For this review, take the finished solid that the model builds, in its own axes (mm). Face numbers are marked on the shaded views. A direction names the side the tool comes from. Round coordinates to 2 decimals unless told otherwise and drop trailing zeros. Write each loop counter-clockwise with the first axis right and the second up, starting at its lowest first coordinate (ties: lowest second). Pieces come first, ordered by that corner, then holes. Notation, with made-up numbers: (25.25, -13.75) -> (57.25, -13.75) arc R21 cw to (57.25, -2.75) -> close; hole circle Ø8 at (47.25, 79). An arc over 180 degrees is marked (long way). Answer as CSV lines item,"result". Start each with the question number.
Item 1: Take a section at B-B on z = 5.75. Give the boundary of the cut face in (x, y), then the cut area to 3 significant figures.
Item 2: Take a section at A-A on y = -2. Give the boundary of the cut face in (x, z).
Item 3: Mouldability with a two-part tool opening along Y and no side actions: class the marked faces 4, 5 and 6 as +Y half, -Y half, draft (parallel to the pull), parting line (faces both ways), or undercut.
Item 4: For pin 1 Ø1.7 at (x, y) = (-17, -1) entering from +Z; pin 2 Ø0.6 at (y, z) = (0, 9) entering from +X; pin 3 Ø4 at (x, y) = (-13, 2) entering from +Z, all flat-tipped, find the tip position at first contact; note any pin that passes through.
Item 5: Take a section at C-C on x = -17. Give the boundary of the cut face in (y, z).
Item 6: Machinability: for the marked faces 1, 2 and 3, which of the approach directions +Z, -Z, +X, -X, +Y, -Y give a long, thin tool a straight path to every point of the face, cutting with its end or side? Answer none if there is none.
Item 7: Wall thickness on probe 1 along Y at (x, z) = (17, 4.25); probe 2 along Y at (x, z) = (16.5, 3.5); probe 3 along Z at (x, y) = (-9.5, -1): over which ranges is each line inside the solid? List them lowest first. Write a range as from..to.
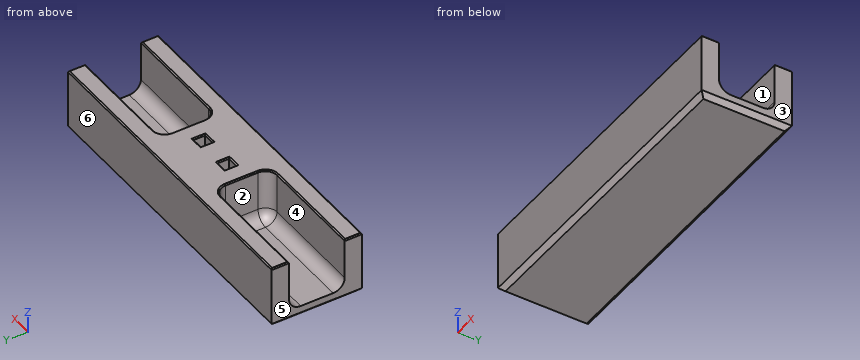
```python
from build123d import *

# Parameters (mm, degrees)
F0_W     = 55
F0_H     = 15.6
F1_DEPTH = 11
F2_W     = 2
F2_H     = 2
F3_DEPTH = 4
F4_W     = 20.27
F4_H     = 9.6
F5_DEPTH = 9
F6_R     = 2
F7_SIZE  = 0.2
F8_SIZE  = 0.8


with BuildPart() as f1:
    # F0 (on Top) → F1 (new body)
    with BuildSketch(Plane.XY):
        Rectangle(F0_W, F0_H)
    extrude(amount=F1_DEPTH)

    # F2 (on face) → F3 (cut)
    with BuildSketch(Plane.XY.offset(11)):
        with Locations((-3.23, 0)):
            Rectangle(F2_W, F2_H)
        with Locations((3.23, 0)):
            Rectangle(F2_W, F2_H)
    extrude(amount=-F3_DEPTH, mode=Mode.SUBTRACT)

    # F4 (on face) → F5 (cut)
    with BuildSketch(Plane.XY.offset(11)):
        with Locations((-17.365, 0)):
            Rectangle(F4_W, F4_H)
        with Locations((17.365, 0)):
            Rectangle(F4_W, F4_H)
    extrude(amount=-F5_DEPTH, mode=Mode.SUBTRACT)

    # F6
    f6_edges = [f1.edges().sort_by_distance(p)[0] for p in [
        (-7.23, 4.8, 6.5),
        (-17.365, 4.8, 2),
        (-7.23, 0, 2),
        (-17.365, -4.8, 2),
        (-7.23, -4.8, 6.5),
        (7.23, 0, 2),
        (7.23, 4.8, 6.5),
        (17.365, 4.8, 2),
        (17.365, -4.8, 2),
        (7.23, -4.8, 6.5),
    ]]
    fillet(f6_edges, radius=F6_R)

    # F7
    f7_edges = [f1.edges().sort_by_distance(p)[0] for p in [
        (-18.365, -4.8, 11),
        (-7.815786, -4.214214, 11),
        (-27.5, -6.3, 11),
        (-7.23, 0, 11),
        (0, -7.8, 11),
        (-7.815786, 4.214214, 11),
        (27.5, -6.3, 11),
        (-18.365, 4.8, 11),
        (18.365, -4.8, 11),
        (-27.5, 6.3, 11),
        (7.815786, -4.214214, 11),
        (0, 7.8, 11),
        (7.23, 0, 11),
        (27.5, 6.3, 11),
        (7.815786, 4.214214, 11),
        (18.365, 4.8, 11),
        (-2.23, 0, 11),
        (-3.23, -1, 11),
        (-3.23, 1, 11),
        (-4.23, 0, 11),
        (3.23, 1, 11),
        (4.23, 0, 11),
        (2.23, 0, 11),
        (3.23, -1, 11),
    ]]
    chamfer(f7_edges, length=F7_SIZE)

    # F8
    f8_edges = [f1.edges().sort_by_distance(p)[0] for p in [
        (27.5, 0, 0),
        (0, 7.8, 0),
        (-27.5, 0, 0),
        (0, -7.8, 0),
    ]]
    chamfer(f8_edges, length=F8_SIZE)


solid = f1.part
```
Output values:
1,outline,"(-27.5, -7.8) -> (27.5, -7.8) -> (27.5, -4.8) -> (9.23, -4.8) arc R2 cw to (7.23, -2.8) -> (7.23, 2.8) arc R2 cw to (9.23, 4.8) -> (27.5, 4.8) -> (27.5, 7.8) -> (-27.5, 7.8) -> (-27.5, 4.8) -> (-9.23, 4.8) arc R2 cw to (-7.23, 2.8) -> (-7.23, -2.8) arc R2 cw to (-9.23, -4.8) -> (-27.5, -4.8) -> close"
1,area,"472 mm^2"
2,outline,"(-27.5, 0.8) -> (-26.7, 0) -> (26.7, 0) -> (27.5, 0.8) -> (27.5, 2) -> (9.23, 2) arc R2 cw to (7.23, 4) -> (7.23, 10.8) -> (7.03, 11) -> (-7.03, 11) -> (-7.23, 10.8) -> (-7.23, 4) arc R2 cw to (-9.23, 2) -> (-27.5, 2) -> close"
3,face 4,"undercut"
3,face 5,"draft"
3,face 6,"+Y half"
4,pin 1,"stops at z = 2"
4,pin 2,"stops at x = 7.23"
4,pin 3,"stops at z = 2.4"
5,outline,"(-7.8, 0.8) -> (-7, 0) -> (7, 0) -> (7.8, 0.8) -> (7.8, 10.8) -> (7.6, 11) -> (5, 11) -> (4.8, 10.8) -> (4.8, 4) arc R2 cw to (2.8, 2) -> (-2.8, 2) arc R2 cw to (-4.8, 4) -> (-4.8, 10.8) -> (-5, 11) -> (-7.6, 11) -> (-7.8, 10.8) -> close"
6,face 1,"+Z, +X"
6,face 2,"+Z, -X"
6,face 3,"+Z, -Z, +X, +Y, -Y"
7,probe 1,"y = -7.8..-4.8, 4.8..7.8"
7,probe 2,"y = -7.8..-4.74, 4.74..7.8"
7,probe 3,"z = 0..2"
